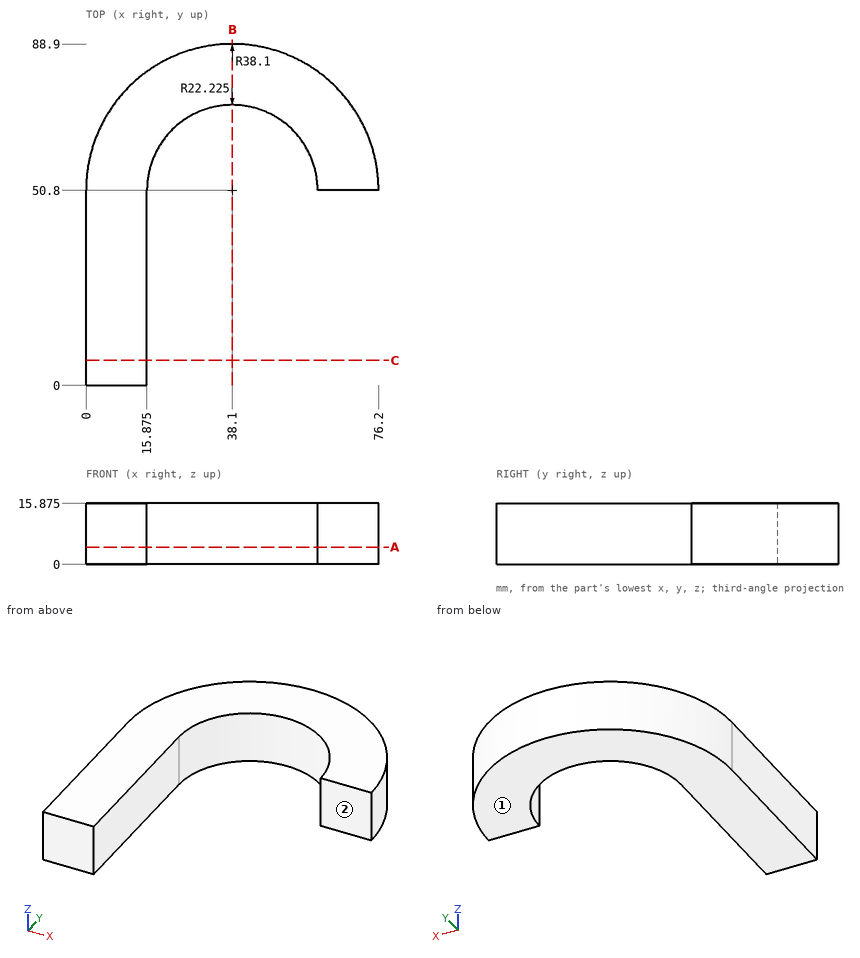
Geometry check sheet. Reference: drawing and pictorial views, mm from the part's lowest x, y, z. A direction names the side the tool comes from. Coordinates: 2 decimals unless noted, no trailing zeros. Order: outer loops, then holes, each group sorted by start corner. A loop starts at its lowest first (then second) coordinate and runs counter-clockwise, first axis right, second up. Notation, with made-up numbers: (29.25, 20.5) - (88.25, 20.5) arc R16 cw to (88.25, 42.5) - close; hole circle Ø2 at (46.25, 85). An arc over 180 degrees is marked (long way). Answer in a Markdown table with one row per item. Add a question column.
1) Material ranges on line 1 along X through (y, z) = (4.5, 11.75) (3 decimals); line 2 along X through (y, z) = (55.5, 9.75); line 3 along X through (y, z) = (68, 8.25), recorded low to high. Write a range as [from, to].
2) Cross-section at B-B, the plane x = 38.1. Record the cut outline in (y, z) (3 decimals), then the cut area to 3 significant figures.
3) Set-up check for the marked faces 1 and 2: record each of +Z, -Z, +X, -X, +Y, -Y from which the full face is reachable in a straight line by a thin tool's end or side.
4) Cross-section at A-A, the plane z = 4.5. Record the cut outline in (x, y) (3 decimals), then the cut area to 3 significant figures.
5) Cross-section at C-C, the plane y = 6.5. Record the cut outline in (x, z) (3 decimals), then the cut area to 3 significant figures.
6) Gauge pin test, flat ends, axial feed: P1, Ø4, axis at y = 47, z = 7, coming from the +X side (3 decimals); P2, Ø4, axis at x = 32, z = 9.5, coming from the +Y side; P3, Ø5, axis at x = 28.5, z = 3, coming from the -Y side; P4, Ø1.5, axis at x = 17.5, y = 39.5, coming from the -Z side. Record the tip position at first contact, or that the pin passes through.
Check result:
| question | item | result |
|---|---|---|
| 1 | line 1 | x = [0, 15.875] |
| 1 | line 2 | x = [0.29, 16.38], [59.82, 75.91] |
| 1 | line 3 | x = [4.1, 24.02], [52.18, 72.1] |
| 2 | outline | (73.025, 0) - (88.9, 0) - (88.9, 15.875) - (73.025, 15.875) - close |
| 2 | area | 252 mm² |
| 3 | face 1 | -Z, +X, -X, +Y, -Y |
| 3 | face 2 | +Z, -Z, +X, -Y |
| 4 | outline | (0, 0) - (15.875, 0) - (15.875, 50.8) arc R22.225 cw to (60.325, 50.8) - (76.2, 50.8) arc R38.1 ccw to (0, 50.8) - close |
| 4 | area | 2,310 mm² |
| 5 | outline | (0, 0) - (15.875, 0) - (15.875, 15.875) - (0, 15.875) - close |
| 5 | area | 252 mm² |
| 6 | P1 | stops at x = 15.875 |
| 6 | P2 | stops at y = 88.68 |
| 6 | P3 | stops at y = 69.44 |
| 6 | P4 | passes through |
